Here's how the part is built. I have some questions about the finished solid (model axes, mm). Face numbers are marked on the shaded views. A direction names the side the tool comes from. Coordinates: 2 decimals unless noted, no trailing zeros. Loops run counter-clockwise (first coordinate to the right, second up) from the corner with the lowest first, then second, coordinate; pieces in that order, holes last. Notation, with made-up numbers: (-35.75, -14.75) -> (12.25, -14.75) arc R16 cw to (12.25, -1.75) -> close; hole circle Ø1 at (26.25, -40). An arc over 180 degrees is marked (long way). Answer as a JSON object with one key per item and string values. Group by question number.
1) If we mould it in two halves opening along X, with no side actions, what happens to the marked faces 1 and 2? For each: +X half, -X half, draft (parallel to the pull), parting line (faces both ways), or undercut.
2) I want a section at D-D (y = 35.5). Write out the boundary of the cut face in (x, z) (3 decimals).
3) I'm going to push flat-ended pins straight in: pin 1 (1.5 mm diameter, centred on y = -10, z = 1, fed in from -X); pin 2 (2 mm diameter, centred on x = 14, z = 2, fed in from +Y). Where does each tip first touch, or does it pass through?
4) I want a section at C-C (x = -39.5). Write out the boundary of the cut face in (y, z) (3 decimals).
5) I need wall thicknesses on probe 1 along Y at (x, z) = (-3, 2.75); probe 2 along Y at (x, z) = (5, 5.5); probe 3 along X at (y, z) = (13.5, 1.75). Which ranges of each line are inside material? Lowest first, please. Write a range as [from, to].
6) I want a section at A-A (z = 3.25). Write out the boundary of the cut face in (x, y), then the cut area to 3 significant figures.
7) I want a section at B-B (y = 3). Write out the boundary of the cut face in (x, z).
8) Which directions (+Z, -Z, +X, -X, +Y, -Y) give clear straight access to the entire face, cutting with the end or side of a thin tool? Please do the marked faces 3, 4 and 5.
```python
from build123d import *

# Parameters (mm, degrees)
F0_R     = 11.15
F1_DEPTH = 7


# Not quite as in the source:
# - a feature names something its author has since deleted; it is built from what else it names


with BuildPart() as f1:
    # F0 (on Top) → F1 (new body)
    with BuildSketch(Plane.XY):
        with BuildLine():
            ThreePointArc((-12.6572045799, -3.5661845468), (-12.883564121, 2.6336809867), (-10.2422641065, 8.2473344769))
            Line((-10.2422641065, 8.2473344769), (-26.0292641065, 8.2473344769))
            ThreePointArc((-26.0292641065, 8.2473344769), (-34.9143148349, 9.7844703454), (-42.7665638646, 14.217200689))
            ThreePointArc((-42.7665638646, 14.217200689), (-39.5806592619, -28.3580220296), (0, -44.3633645773))
            ThreePointArc((0, -44.3633645773), (-15.7763325785, -26.6479576979), (-21.2499108166, -3.5661845468))
            Line((-21.2499108166, -3.5661845468), (-12.6572045799, -3.5661845468))
        make_face()
        with BuildLine():
            ThreePointArc((12.9567624843, -2.2460645415), (13.1016015561, -1.1271808486), (13.15, 0))
            ThreePointArc((13.15, 0), (12.2942286487, 4.6663092411), (9.8382978048, 8.7252734229))
            ThreePointArc((9.8382978048, 8.7252734229), (-0.3128955133, 13.1462769025), (-10.2422641065, 8.2473344769))
            ThreePointArc((-10.2422641065, 8.2473344769), (-12.883564121, 2.6336809867), (-12.6572045799, -3.5661845468))
            ThreePointArc((-12.6572045799, -3.5661845468), (0.6768404107, -13.1325697051), (12.9567624843, -2.2460645415))
        make_face()
        Circle(F0_R, mode=Mode.SUBTRACT)
        with BuildLine():
            ThreePointArc((9.8382978048, 8.7252734229), (12.2942286487, 4.6663092411), (13.15, 0))
            ThreePointArc((13.15, 0), (13.1016015561, -1.1271808486), (12.9567624843, -2.2460645415))
            Line((12.9567624843, -2.2460645415), (28.7434491243, -2.2460645415))
            ThreePointArc((28.7434491243, -2.2460645415), (35.3157092291, -3.6070761232), (40.8069513167, -7.4662490586))
            ThreePointArc((40.8069513167, -7.4662490586), (38.839648653, 33.6212574976), (0, 47.1687726676))
            ThreePointArc((0, 47.1687726676), (16.0453137764, 31.2214280727), (18.4312978048, 8.7252734229))
            Line((18.4312978048, 8.7252734229), (9.8382978048, 8.7252734229))
        make_face()
    extrude(amount=F1_DEPTH)


solid = f1.part
```
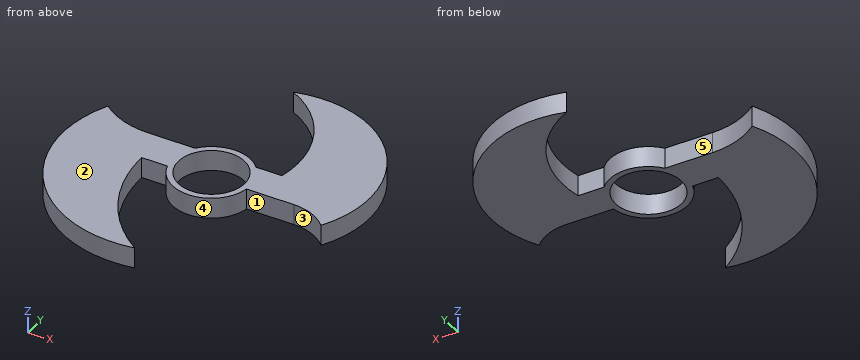
Determined:
{
 "1": {"face 1": "undercut", "face 2": "draft"},
 "2": {"outline": "(13.595, 0) -> (37.338, 0) -> (37.338, 7) -> (13.595, 7) -> close"},
 "3": {"pin 1": "x = -47.08", "pin 2": "y = 48.21"},
 "4": {"outline": "(-28.468, 0) -> (11.935, 0) -> (11.935, 7) -> (-28.468, 7) -> close"},
 "5": {"probe 1": "[-44.77, -42.16], [-12.8, -10.74], [10.74, 12.8]", "probe 2": "[-12.16, -9.97], [9.97, 12.16], [44.26, 48.12]", "probe 3": "[-43.13, -41.85], [19.22, 46.1]"},
 "6": {"outline": "(-42.77, 14.22) arc R40.45 ccw to (0, -44.36) arc R48.44 cw to (-21.25, -3.57) -> (-12.66, -3.57) arc R13.15 ccw to (12.96, -2.25) -> (28.74, -2.25) arc R16.55 cw to (40.81, -7.47) arc R36.77 ccw to (0, 47.17) arc R33.78 cw to (18.43, 8.73) -> (9.84, 8.73) arc R13.15 ccw to (-10.24, 8.25) -> (-26.03, 8.25) arc R26.45 cw to start; hole circle Ø22.3 at (0, 0)", "area": "2,940 mm^2"},
 "7": {"outline": "(-46.66, 0) -> (-10.74, 0) -> (-10.74, 7) -> (-46.66, 7) -> close; (10.74, 0) -> (45.12, 0) -> (45.12, 7) -> (10.74, 7) -> close"},
 "8": {"face 3": "+Z, -Z, -Y", "face 4": "+Z, -Z", "face 5": "+Z, -Z, +Y"}
}
